from build123d import *

# Parameters (mm, degrees)
SKETCH1_R           = 2.9337
BOSS_EXTRUDE1_DEPTH = 190.5


with BuildPart() as part:
    # Sketch1 → Boss-Extrude1 (new body)
    with BuildSketch(Plane.XY.offset(304.8)):
        with BuildLine():
            Line((6.293011699, -1.800184894), (7.332348803, -2.22e-07))
            Line((7.332348803, -2.22e-07), (6.293011439, 1.800184522))
            ThreePointArc((6.293011439, 1.800184522), (4.124446058, 2.381249653), (4.705511189, 4.549815034))
            Line((4.705511189, 4.549815034), (3.666173825, 6.349999778))
            Line((3.666173825, 6.349999778), (1.587499615, 6.349999778))
            ThreePointArc((1.587499615, 6.349999778), (-3.85e-07, 4.762499778), (-1.587500385, 6.349999778))
            Line((-1.587500385, 6.349999778), (-3.666174594, 6.349999778))
            Line((-3.666174594, 6.349999778), (-4.70551159, 4.549815043))
            ThreePointArc((-4.70551159, 4.549815043), (-4.12444613, 2.38124975), (-6.293011423, 1.80018429))
            Line((-6.293011423, 1.80018429), (-7.332348419, -4.44e-07))
            Line((-7.332348419, -4.44e-07), (-6.293011205, -1.800185053))
            ThreePointArc((-6.293011205, -1.800185053), (-4.124445841, -2.38125025), (-4.705511038, -4.549815614))
            Line((-4.705511038, -4.549815614), (-3.666173825, -6.350000222))
            Line((-3.666173825, -6.350000222), (-1.587499615, -6.350000222))
            ThreePointArc((-1.587499615, -6.350000222), (3.85e-07, -4.762500222), (1.587500385, -6.350000222))
            Line((1.587500385, -6.350000222), (3.666174594, -6.350000222))
            Line((3.666174594, -6.350000222), (4.705511699, -4.549815551))
            ThreePointArc((4.705511699, -4.549815551), (4.12444637, -2.381250222), (6.293011699, -1.800184894))
        make_face()
        with Locations(Location((0, 0, 0), (0, 0, 180))):
            Circle(SKETCH1_R, mode=Mode.SUBTRACT)
    extrude(amount=-BOSS_EXTRUDE1_DEPTH)


solid = part.part
Geometry: final body of the model. Coordinates: model frame, mm. Give positions to 0.01 mm unless a question says otherwise; leave off trailing zeros. Write each loop counter-clockwise with the first axis right and the second up, starting at its lowest first coordinate (ties: lowest second). Pieces come first, ordered by that corner, then holes. Notation, with made-up numbers: (-27.5, -33) -> (31.5, -33) arc R6 cw to (31.5, -27) -> close; hole circle Ø2 at (-10, 10.25). An arc over 180 degrees is marked (long way). Answer in a Markdown table with one row per item.
(1) Pin query (flat end, axial travel): pin 1 (3 mm diameter, centred on y = 2, z = 148.5, fed in from +X); pin 2 (4.5 mm diameter, centred on x = 0, y = 0, fed in from +Z); pin 3 (1 mm diameter, centred on y = -3, z = 255.5, fed in from +X); pin 4 (3 mm diameter, centred on y = 3.5, z = 140.5, fed in from -X). Return the tip coordinate at first contact, or that it passes through.
Answers below:
| item | result |
|---|---|
| pin 1 | x = 7.04 |
| pin 2 | through |
| pin 3 | x = 4.06 |
| pin 4 | x = -4.71 |
(2) Ray query, line 1 along Y through (x, z) = (0, 258); line 2 along Y through (x, z) = (-4.5, 129); line 3 along Y through (x, z) = (-2, 167.5). Return the intervals inside material, ascending. Write a range as [from, to].
Answers below:
| item | result |
|---|---|
| line 1 | [-4.76, -2.93], [2.93, 4.76] |
| line 2 | [-4.91, -4.41], [-1.94, 1.94], [4.41, 4.91] |
| line 3 | [-6.35, -2.15], [2.15, 6.35] |
(3) Section query A-A on x = 0. Return loops of the section in (y, z).
Answers below:
| item | result |
|---|---|
| outline | (-4.76, 114.3) -> (-2.93, 114.3) -> (-2.93, 304.8) -> (-4.76, 304.8) -> close; (2.93, 114.3) -> (4.76, 114.3) -> (4.76, 304.8) -> (2.93, 304.8) -> close |
(4) Draft query along X for faces 1 (the cylindrical face through (4.142, 2.351, 210.884)), 2 (the flat face through (3.2, 0.1, 114.3)). Return one class per face: +X half, -X half, draft (parallel to the pull), parting line (faces both ways), or undercut.
Answers below:
| item | result |
|---|---|
| face 1 | undercut |
| face 2 | draft |
